Design review of the part built by this model. Coordinates are the model's own, in mm. A direction names the side the tool comes from. Round coordinates to 2 decimals unless told otherwise and drop trailing zeros. Write each loop counter-clockwise with the first axis right and the second up, starting at its lowest first coordinate (ties: lowest second). Pieces come first, ordered by that corner, then holes. Notation, with made-up numbers: M 77,-2 L 120,-2 A21 cw 120,24 Z; hole C 52.5,87 d2. An arc over 180 degrees is marked long. One line per question, with ' | ' between items. Start each with the question number.
Item 1: Insertion check: pin 1 Ø0.9 at (y, z) = (2, -33.5) entering from -X; pin 2 Ø1 at (x, y) = (31.5, 1) entering from -Z; pin 3 Ø1 at (x, y) = (25, 2) entering from +Z; pin 4 Ø3 at (x, z) = (-57.61, 57) entering from +Y. Each pin has a flat end and moves straight along its axis. Give the tip position at first contact, or say it passes through.
Item 2: Draft analysis for pull direction Z (two halves, no side actions). For faces 6 (the face through (-58, 1, 61)), 7 (the face through (58, 1, -61)), 8 (the face through (56.11, 1, 0)), state which applies: released by +Z, released by -Z, zero draft, split by the parting line, or undercut.
Item 3: Add section A-A, the plane z = -57. State the section outline as (x, y) points.
Item 4: Add section D-D, the plane z = 10. State the section outline as (x, y) points.
Item 5: Add section B-B, the plane z = -27. State the section outline as (x, y) points, and give its area (3 significant figures).
Item 6: Add section C-C, the plane x = -9.5. State the section outline as (y, z) points, and give its area (3 significant figures).
Item 7: For L1, parallel to X at y = 1.4, z = 47; L2, parallel to Z at x = 10, y = 1.7; L3, parallel to Z at x = 23.5, y = 1.9, list the stretches that pass through material, from the lowest coordinate up.
Item 8: Machinability: for faces 1 (the face through (-56.11, 1, 28)), 2 (the face through (-59.11, 1, 1)), 3 (the face through (-1, 1, 58.5)), 4 (the face through (-61.61, 1, -57)), 5 (the face through (1, 0, 1)), which of the approach directions +Z, -Z, +X, -X, +Y, -Y give a long, thin tool a straight path to every point of the face, cutting with its end or side? Answer none if there is none.
Autodesk Inventor part; units mm, degrees
ref_plane "YZ Plane" through (0, 0, 0) normal (1, 0, 0) x (0, 1, 0)
ref_plane "XZ Plane" through (0, 0, 0) normal (0, 1, 0) x (-1, 0, 0)
ref_plane "XY Plane" through (0, 0, 0) normal (0, 0, 1) x (1, 0, 0)
sketch "Sketch1" plane through (0, 0, 0) normal (0, 1, 0) x (-1, 0, 0)
  line L0 (75, 65) -> (-75, 65)
  line L1 (-75, 65) -> (-75, -65)
  line L2 (-75, -65) -> (75, -65)
  line L3 (75, -65) -> (75, 65)
  line L4 (75, 65) -> (-75, -65) construction
  line L5 (-75, 65) -> (75, -65) construction
  line L6 (62.0096, 65) -> (62.0096, -65)
  line L7 (105, 0) -> (-105, 0)
  line L8 (0, -91) -> (0, 91)
  line L9 (-62.0096, 65) -> (-62.0096, -65)
  line L10 (61.6096, 65) -> (61.6096, -65)
  line L11 (-61.6096, 65) -> (-61.6096, -65)
  line L12 (-71, 61) -> (71, 61)
  line L13 (71, 61) -> (71, -61)
  line L14 (71, -61) -> (-71, -61)
  line L15 (-71, -61) -> (-71, 61)
  line L16 (61.6096, 61) -> (53.6096, 61)
  line L17 (53.6096, 61) -> (53.6096, 53)
  line L18 (53.6096, 53) -> (61.6096, 53)
  line L19 (61.6096, 53) -> (61.6096, 61)
  line L20 (61.6096, -61) -> (53.6096, -61)
  line L21 (53.6096, -61) -> (53.6096, -53)
  line L22 (53.6096, -53) -> (61.6096, -53)
  line L23 (-61.6096, 61) -> (-53.6096, 61)
  line L24 (-53.6096, 61) -> (-53.6096, 53)
  line L25 (-53.6096, 53) -> (-61.6096, 53)
  line L26 (-61.6096, 53) -> (-61.6096, 61)
  line L27 (-53.6096, -61) -> (-53.6096, -53)
  line L28 (-53.6096, -53) -> (-61.6096, -53)
  line L29 (-61.6096, -61) -> (-53.6096, -61)
  line L30 (-61.6096, 12) -> (-53.6096, 12)
  line L31 (-53.6096, 12) -> (-53.6096, 20)
  line L32 (-53.6096, 20) -> (-61.6096, 20)
  line L33 (-61.6096, 20) -> (-61.6096, 12)
  line L34 (-61.6096, -12) -> (-53.6096, -12)
  line L35 (-53.6096, -12) -> (-53.6096, -20)
  line L36 (-53.6096, -20) -> (-61.6096, -20)
  circle A0 centre (57.6096, 57) radius 1.55
  line L37 (61.6096, 57) -> (53.6096, 57)
  line L38 (57.6096, 61) -> (57.6096, 53)
  circle A1 centre (57.6096, -57) radius 1.55
  circle A2 centre (-57.6096, 57) radius 1.55
  circle A3 centre (-57.6096, -57) radius 1.55
  line L39 (-53.6096, 16) -> (-61.6096, 16)
  line L40 (-57.6096, 20) -> (-57.6096, 12)
  circle A4 centre (-57.6096, 16) radius 1.55
  circle A5 centre (-57.6096, -16) radius 1.55
  line L41 (53.6096, 57) -> (-53.6096, 57)
  line L42 (57.6096, 53) -> (57.6096, -53)
  line L43 (53.6096, -57) -> (-53.6096, -57)
  line L44 (-57.6096, -53) -> (-57.6096, -20)
  line L45 (-57.6096, -12) -> (-57.6096, 12)
  line L46 (-57.6096, 20) -> (-57.6096, 53)
  line L47 (53.6096, 53) -> (-53.6096, -53)
  line L48 (-53.6096, 53) -> (53.6096, -53)
  line L49 (0, 0) -> (57.6096, 0)
  line L50 (0, 0) -> (-57.6096, 0)
  line L51 (0, 0) -> (-53.6096, 16)
  line L52 (0, 0) -> (-53.6096, -16)
  circle A6 centre (0, 0) radius 6
  line L53 (53.6096, 55.1093) -> (3.0768, 5.1511)
  line L54 (53.6096, 58.5) -> (-53.6096, 58.5)
  line L55 (59.1096, 53) -> (59.1096, -53)
  line L56 (53.6096, -58.5) -> (-53.6096, -58.5)
  line L57 (-59.1096, -53) -> (-59.1096, -20)
  line L58 (-59.1096, -12) -> (-59.1096, 12)
  line L59 (-59.1096, 20) -> (-59.1096, 53)
  line L60 (-55.7432, 53) -> (-5.1859, 3.0177)
  line L61 (-5.9958, 0.2241) -> (-53.6096, 14.4346)
  line L62 (-53.6096, -17.5654) -> (-5.1378, -3.0988)
  line L63 (-3.0768, -5.1511) -> (-53.6096, -55.1093)
  line L64 (5.8095, -1.5) -> (57.6096, -1.5)
  line L65 (56.1096, 53) -> (56.1096, -53)
  line L66 (53.6096, 55.5) -> (-53.6096, 55.5)
  line L67 (55.7188, 52.9759) -> (5.1859, 3.0177)
  line L68 (5.8095, 1.5) -> (57.6096, 1.5)
  line L69 (-53.634, 55.1334) -> (-3.0768, 5.1511)
  line L70 (-5.1378, 3.0988) -> (-52.7517, 17.3093)
  line L71 (-5.1859, -3.0177) -> (-55.7188, -52.9759)
  line L72 (53.6096, -55.5) -> (-53.6096, -55.5)
  line L73 (-56.1096, -53) -> (-56.1096, -20)
  line L74 (-56.1096, -12) -> (-56.1096, 12)
  line L75 (-56.1096, 20) -> (-56.1096, 53)
  line L76 (-54.4676, -14.6907) -> (-5.9958, -0.2241)
  line L77 (3.0768, -5.1511) -> (53.6096, -55.1093)
  line L78 (5.1859, -3.0177) -> (55.7188, -52.9759)
  line L79 (1.5, 55.5) -> (1.5, 5.8095)
  line L80 (-1.5, 55.5) -> (-1.5, 5.8095)
  line L81 (1.5, -55.5) -> (1.5, -5.8095)
  line L82 (-1.5, -55.5) -> (-1.5, -5.8095)
  line L83 (-52.7517, 17.3093) -> (-53.6096, 17.5654)
  line L84 (55.7188, -52.9759) -> (55.7432, -53)
  line L85 (55.7188, 52.9759) -> (55.7432, 53)
  line L86 (-55.7188, -52.9759) -> (-55.7432, -53)
  point P0 (-61.6096, 61)
  point P1 (-61.6096, 0)
  point P2 (-71, 0)
  point P3 (4.2668, -4.2183)
  point P4 (56.1096, -1.5)
  point P5 (-4.2668, -4.2183)
  point P6 (-56.1096, -20)
  point P7 (1.5, -5.8095)
  point P8 (-1.5, -5.8095)
  point P9 (-1.5, 5.8095)
  point P10 (-3.0768, 5.1511)
  point P11 (-53.6096, 55.1093)
  point P12 (56.1096, 1.5)
  point P13 (4.2668, 4.2183)
  point P14 (-53.6096, -14.4346)
  point P15 (-5.7494, 1.7159)
  point P16 (-61.6096, -61)
  point P17 (61.6096, -61)
  point P18 (-5.3243, -3.1544)
  point P19 (5.1859, 3.0177)
  point P20 (-5.3243, 3.1544)
  dimension "d13" = 12
  dimension "d0" = 150
  dimension "d1" = 130
  dimension "d2" = 12.9904
  dimension "d3" = 0.4
  dimension "d4" = 4
  dimension "d5" = 8
  dimension "d6" = 8
  dimension "d7" = 8
  dimension "d8" = 8
  dimension "d9" = 12
  dimension "d10" = 3.1
  dimension "d11" = 3.1
  dimension "d14" = 3
  dimension "d15" = 3
  dimension "d16" = 3
  dimension "d17" = 3
  dimension "d18" = 3
  dimension "d19" = 3
  dimension "d20" = 3
  dimension "d21" = 3
  dimension "d22" = 3
  dimension "d23" = 3
  dimension "d24" = 3
  dimension "d25" = 3
extrude "Extrusion1" add sketch "Sketch1" along normal blind 3 contours L10 L37 A0 L38 L12 | L10 L18 L38 A0 L37 | L38 A0 L37 L17 L12 | L12 L24 L25 L11 | L54 L17 L41 L8 | L8 L41 L24 L54 | L14 L21 L22 L10 | L55 L22 L42 L7 | L7 L42 L18 L55 | L41 L17 L66 L8 | L8 L66 L24 L41 | L38 L18 L17 L37 A0 | L42 L64 L65 L7 | L7 L65 L68 L42 | L32 L40 A4 L39 L11 | L25 L46 L32 L59 | L66 L79 A6 L8 | L8 A6 L80 L66 | L42 L68 L65 L18 | L56 L8 L43 L21 | L65 L64 A6 L7 | L7 A6 L68 L65 | L42 L22 L65 L64 | L11 L28 L27 L14 | L56 L27 L43 L8 | L39 A4 L40 L30 L11 | L25 L75 L32 L46 | A6 L47 L8 | L8 L48 A6 | L43 L8 L72 L21 | A6 L48 L7 | L7 L47 A6 | L43 L27 L72 L8 | L58 L30 L45 L7 | L7 L45 L34 L58 | L34 L35 L36 L11 | L32 L31 L39 A4 L40 | L52 A6 L7 | L48 A6 L8 | L8 A6 L47 | L51 A6 L48 | L7 A6 L51 | L47 A6 L52 | L17 L47 A6 L53 | L69 A6 L48 L24 | L85 L67 A6 L47 L18 | L22 L48 A6 L78 L84 | L57 L36 L44 L28 | L72 L82 A6 L8 | L8 A6 L81 L72 | L45 L30 L74 L7 | L7 L74 L34 L45 | A4 L39 L31 L30 L40 | L25 L48 A6 L70 L60 | A6 L63 L27 L47 | L47 L28 L86 L71 L62 A6 | L48 L21 L77 A6 | A6 L61 L31 L51 | L51 L31 L83 L70 L60 A6 | A6 L71 L62 L35 L52 | L52 L35 L76 A6 | L44 L36 L73 L28 | L70 A6 L60 | L62 L71 A6
equation "\"d0\" = BodyLength"
equation "\"d1\" = BodyWidth"
equation "\"d2\" = 0.433013 * BodyHeight"
equation "\"d4\" = SideThickness"
equation "\"d5\" = M3ScrewInsertBrim"
equation "\"d6\" = M3ScrewInsertBrim"
equation "\"d7\" = M3ScrewInsertBrim"
equation "\"d8\" = M3ScrewInsertBrim"
equation "\"d10\" = M3ScrewDia"
equation "\"d11\" = M3ScrewDia"
properties part number "HexScrewGuide"
Computed values:
1) pin 1: stops at x = -59.11 | pin 2: stops at z = -58.5 | pin 3: stops at z = 58.5 | pin 4: passes through
2) face 6: released by +Z | face 7: released by -Z | face 8: undercut
3) outline: M -61.61,0 L -59.16,0 L -59.16,3 L -61.61,3 Z; M -56.06,0 L 56.06,0 L 56.06,3 L -56.06,3 Z; M 59.16,0 L 61.61,0 L 61.61,3 L 59.16,3 Z
4) outline: M -59.11,0 L -56.11,0 L -56.11,3 L -59.11,3 Z; M -12.25,0 L -7.98,0 L -7.98,3 L -12.25,3 Z; M -1.5,0 L 1.5,0 L 1.5,3 L -1.5,3 Z; M 7.98,0 L 12.25,0 L 12.25,3 L 7.98,3 Z; M 28.26,0 L 38.75,0 L 38.75,3 L 28.26,3 Z; M 56.11,0 L 59.11,0 L 59.11,3 L 56.11,3 Z
5) outline: M -59.11,0 L -56.11,0 L -56.11,3 L -59.11,3 Z; M -29.44,0 L -25.18,0 L -25.18,3 L -29.44,3 Z; M -1.5,0 L 1.5,0 L 1.5,3 L -1.5,3 Z; M 25.18,0 L 29.44,0 L 29.44,3 L 25.18,3 Z; M 56.11,0 L 59.11,0 L 59.11,3 L 56.11,3 Z | area: 52.6 mm^2
6) outline: M 0,-58.5 L 3,-58.5 L 3,-55.5 L 0,-55.5 Z; M 0,-11.5 L 3,-11.5 L 3,-7.28 L 0,-7.28 Z; M 0,-1.5 L 3,-1.5 L 3,1.5 L 0,1.5 Z; M 0,7.28 L 3,7.28 L 3,11.5 L 0,11.5 Z; M 0,55.5 L 3,55.5 L 3,58.5 L 0,58.5 Z | area: 52.3 mm^2
7) L1: x = -59.11 to -56.11, -49.67 to -45.41, -1.5 to 1.5, 45.41 to 49.67, 56.11 to 59.11 | L2: z = -58.5 to -55.5, -12 to -7.78, -4.55 to -1.42, 1.42 to 4.55, 7.78 to 12, 55.5 to 58.5 | L3: z = -58.5 to -55.5, -25.34 to -21.12, -8.58 to -5.45, 5.45 to 8.58, 21.12 to 25.34, 55.5 to 58.5
8) face 1: +Y, -Y | face 2: -X, +Y, -Y | face 3: +Z, +Y, -Y | face 4: +Z, -Z, -X, +Y, -Y | face 5: +Z, -Z, +X, -X, -Y
